Verification items for this drawing (mm, ordinates from the low corner). Coordinates: 2 decimals unless noted, no trailing zeros. Loops run counter-clockwise (first coordinate to the right, second up) from the corner with the lowest first, then second, coordinate; pieces in that order, holes last. Notation, with made-up numbers: (62.5, 62) -> (94.5, 62) arc R24 ccw to (94.5, 101) -> close; hole circle Ø10 at (28.25, -30.75). An arc over 180 degrees is marked (long way). Write item = value, one per line.
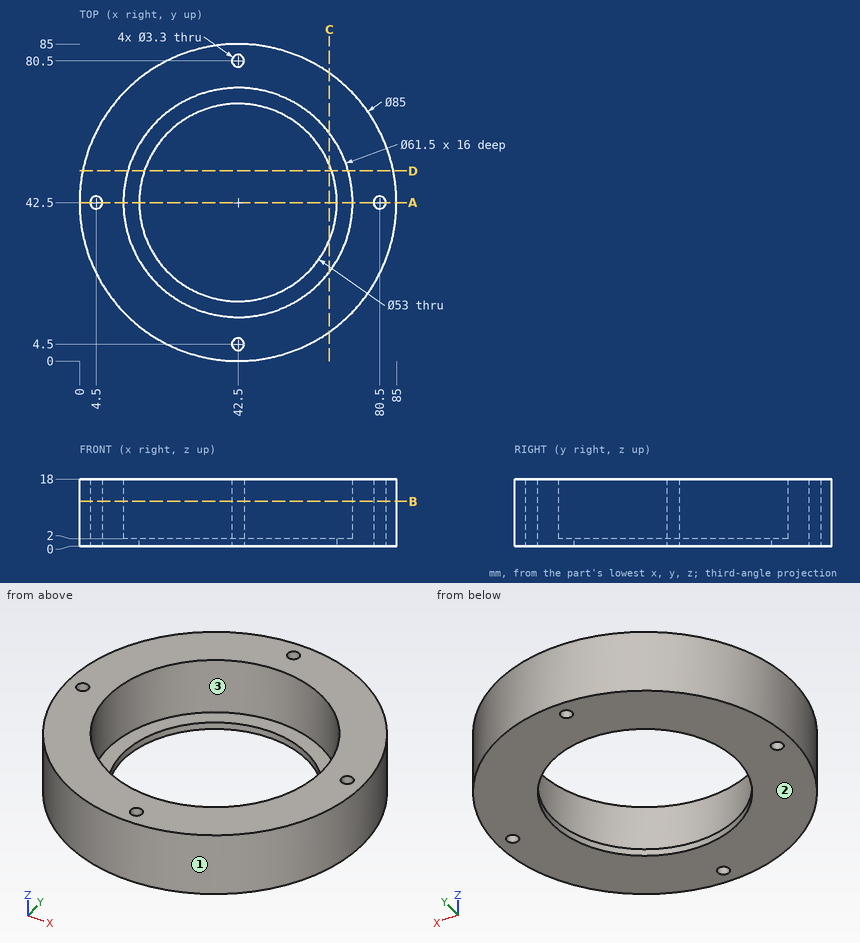
1) Sectioned sample at B-B, the plane z = 12. Record the cut outline in (x, y), plus the area to 3 significant figures.
Ans:
outline = circle Ø85 at (42.5, 42.5); hole circle Ø3.3 at (4.5, 42.5); hole circle Ø61.5 at (42.5, 42.5); hole circle Ø3.3 at (42.5, 4.5); hole circle Ø3.3 at (42.5, 80.5); hole circle Ø3.3 at (80.5, 42.5)
area = 2,670 mm2
2) Sectioned sample at C-C, the plane x = 67. Record the cut outline in (y, z), plus the area to 3 significant figures.
Ans:
outline = (7.77, 0) -> (32.4, 0) -> (32.4, 2) -> (23.92, 2) -> (23.92, 18) -> (7.77, 18) -> close; (52.6, 0) -> (77.23, 0) -> (77.23, 18) -> (61.08, 18) -> (61.08, 2) -> (52.6, 2) -> close
area = 615 mm2
3) Depth check by flat-ended pin: pin 1 Ø4.5 at (x, y) = (42.5, 80.5) entering from +Z; pin 2 Ø2 at (x, z) = (49, 15.5) entering from -Y; pin 3 Ø1 at (y, z) = (44, 10.5) entering from -X; pin 4 Ø8 at (y, z) = (60, 2) entering from -X. Enter the tip coordinate at first touch or a pass-through.
Ans:
pin_1 = 18
pin_2 = 0.36
pin_3 = 0.01
pin_4 = 2.2
4) Sectioned sample at A-A, the plane y = 42.5. Record the cut outline in (x, z), plus the area to 3 significant figures.
Ans:
outline = (0, 0) -> (2.85, 0) -> (2.85, 18) -> (0, 18) -> close; (6.15, 0) -> (16, 0) -> (16, 2) -> (11.75, 2) -> (11.75, 18) -> (6.15, 18) -> close; (69, 0) -> (78.85, 0) -> (78.85, 18) -> (73.25, 18) -> (73.25, 2) -> (69, 2) -> close; (82.15, 0) -> (85, 0) -> (85, 18) -> (82.15, 18) -> close
area = 321 mm2
5) Material ranges on line 1 (Y direction, x = 42.5, z = 11.75); line 2 (Y direction, x = 42.5, z = 1.15); line 3 (Z direction, x = 56.5, y = 67), recorded low to high.
Ans:
line_1 = 0 to 2.85, 6.15 to 11.75, 73.25 to 78.85, 82.15 to 85
line_2 = 0 to 2.85, 6.15 to 16, 69 to 78.85, 82.15 to 85
line_3 = 0 to 2
6) Sectioned sample at D-D, the plane y = 51. Record the cut outline in (x, z), plus the area to 3 significant figures.
Ans:
outline = (0.86, 0) -> (17.4, 0) -> (17.4, 2) -> (12.95, 2) -> (12.95, 18) -> (0.86, 18) -> close; (67.6, 0) -> (84.14, 0) -> (84.14, 18) -> (72.05, 18) -> (72.05, 2) -> (67.6, 2) -> close
area = 453 mm2
7) Release check for a two-part mould opening along X. For the marked faces 1, 2 and 3 record: pulls with the +X half, pulls with the -X half, needs draft (parallel to the pull), parting line crosses it, or undercut.
Ans:
face_1 = parting line crosses it
face_2 = needs draft
face_3 = undercut
